from build123d import *

# Parameters (mm, degrees)
F0_R     = 6.5
F1_DEPTH = 0.95
F3_DEPTH = 3.25
F4_R     = 2.09999
F5_R     = 1.15
F6_DEPTH = 25


# Not quite as in the source:
# - a fillet or chamfer is up to 0.001 mm smaller than in the source, because OpenCascade refuses the exact size


with BuildPart() as f1:
    # F0 (on Top) → F1 (new body)
    with BuildSketch(Plane.XY):
        with BuildLine():
            Line((25.6782327866, 7.4), (28.5, 7.4))
            Line((28.5, 7.4), (28.5, 11.6))
            Line((28.5, 11.6), (25.6782327866, 11.6))
            ThreePointArc((25.6782327866, 11.6), (22.6641990968, 12.0908046465), (19.9615973522, 13.5125050702))
            Line((19.9615973522, 13.5125050702), (15.2166354344, 17.0874949298))
            ThreePointArc((15.2166354344, 17.0874949298), (12.5140336898, 18.5091953535), (9.5, 19))
            ThreePointArc((9.5, 19), (2.7824855787, 16.2175144213), (0, 9.5))
            ThreePointArc((0, 9.5), (2.7824855787, 2.7824855787), (9.5, 0))
            ThreePointArc((9.5, 0), (12.5140336898, 0.4908046465), (15.2166354344, 1.9125050702))
            Line((15.2166354344, 1.9125050702), (19.9615973522, 5.4874949298))
            ThreePointArc((19.9615973522, 5.4874949298), (22.6641990968, 6.9091953535), (25.6782327866, 7.4))
        make_face()
        with Locations((9.5, 9.5)):
            Circle(F0_R, mode=Mode.SUBTRACT)
    extrude(amount=F1_DEPTH)

    # F2 (on face) → F3 (join)
    with BuildSketch(Plane.XY.offset(0.95)):
        Polygon((28.5, 7.4), (28.5, 11.6), (25.6782327866, 11.6), (24, 11.6), (24, 7.4), (25.6782327866, 7.4), align=None)
    extrude(amount=F3_DEPTH)

    # F4 (radius 2.1 in the source; OpenCascade refuses exactly that, so slightly less here)
    f4_edges = [f1.edges().sort_by_distance(p)[0] for p in [
        (26.25, 11.6, 4.2),
        (26.25, 7.4, 4.2),
    ]]
    fillet(f4_edges, radius=F4_R)

    # F5 (on face) → F6 (cut)
    with BuildSketch(Plane.YZ.offset(28.5)):
        with Locations((9.5, 2.1)):
            Circle(F5_R)
    extrude(amount=-F6_DEPTH, mode=Mode.SUBTRACT)


solid = f1.part
Read the model definition and answer for the solid it produces. Units are mm, in the model's axes. A direction names the side the tool comes from. Coordinates: 2 decimals unless noted, no trailing zeros. Loops run counter-clockwise (first coordinate to the right, second up) from the corner with the lowest first, then second, coordinate; pieces in that order, holes last. Notation, with made-up numbers: (-28, 32) -> (21, 32) arc R29 ccw to (21, 59) -> close; hole circle Ø3 at (-5.5, 27). An arc over 180 degrees is marked (long way). Write item = value, one per line. Start each with the question number.
1) The part is cut by section B-B, the plane y = 3.75. Determine the outline of the cut face in (x, z).
2) Find the intervals of material crossed by L1, parallel to Z at x = 25.1, y = 9.5; L2, parallel to Y at x = 25.95, z = 2.1; L3, parallel to Z at x = 1.75, y = 9.5, in increasing order. Write a range as from..to.
3) The part is cut by section A-A, the plane z = 0.5. Determine the outline of the cut face in (x, y).
4) For faces 1 (the face through (22.7, 12.08, 0.47)), 2 (the face through (27, 7.4, 1)), 3 (the face through (24, 10, 3.3)), determine the directions among +Z, -Z, +X, -X, +Y, -Y from which every point of the face is accessible in a straight line to the end or side of a thin tool.
5) The part is cut by section C-C, the plane z = 2.85. Determine the outline of the cut face in (x, y), plus the area to 3 significant figures.
6) The part is cut by section D-D, the plane x = 21. Determine the outline of the cut face in (y, z), plus the area to 3 significant figures.
7) The mould has two halves that part along Z. Classify faces 4 (the face through (26.22, 11, 3.57)), 5 (the face through (26.282, 10.597, 2.445)), 6 (the face through (27, 11.6, 1)): pulls with the +Z half, pulls with the -Z half, needs draft (parallel to the pull), parting line crosses it, or undercut.
8) Given P1, Ø2.5, axis at x = 26.5, z = 1, coming from the -Y side; P2, Ø1.1, axis at x = 26.5, z = 1.5, coming from the +Y side; P3, Ø1.5, axis at y = 7.5, z = 3, coming from the -X side, each flat-ended and moving along its own axis, determine where each tip first touches the part or whether it passes through.
Result:
q1.outline = (1.94, 0) -> (6.47, 0) -> (6.47, 0.95) -> (1.94, 0.95) -> close; (12.53, 0) -> (17.66, 0) -> (17.66, 0.95) -> (12.53, 0.95) -> close
q2.L1 = 0..0.95, 3.25..4.2
q2.L2 = 7.4..8.35, 10.65..11.6
q2.L3 = 0..0.95
q3.outline = (15.22, 1.91) -> (19.96, 5.49) arc R9.5 cw to (25.68, 7.4) -> (28.5, 7.4) -> (28.5, 11.6) -> (25.68, 11.6) arc R9.5 cw to (19.96, 13.51) -> (15.22, 17.09) arc R9.5 ccw (long way) to start; hole circle Ø13 at (9.5, 9.5)
q4.face_1 = +Z, -Z, +X, +Y
q4.face_2 = +Z, +X, -Y
q4.face_3 = +Z, -X, +Y, -Y
q5.outline = (24, 7.54) -> (28.5, 7.54) -> (28.5, 8.63) -> (24, 8.63) -> close; (24, 10.37) -> (28.5, 10.37) -> (28.5, 11.46) -> (24, 11.46) -> close
q5.area = 9.81 mm²
q6.outline = (6.17, 0) -> (12.83, 0) -> (12.83, 0.95) -> (6.17, 0.95) -> close
q6.area = 6.33 mm²
q7.face_4 = pulls with the +Z half
q7.face_5 = undercut
q7.face_6 = needs draft
q8.P1 = 7.39
q8.P2 = 11.6
q8.P3 = 24
